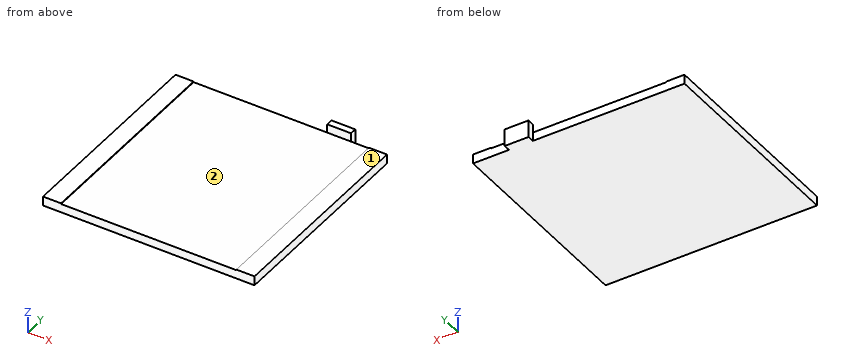
from build123d import *

# Parameters (mm, degrees)
SKETCH1_W           = 159.25
SKETCH1_H           = 155.74
BOSS_EXTRUDE1_DEPTH = 6.5
SKETCH2_W           = 13.61
SKETCH2_H           = 155.74
BOSS_EXTRUDE2_DEPTH = 0.5
SKETCH3_W           = 17.92
SKETCH3_H           = 13
BOSS_EXTRUDE3_DEPTH = 5


with BuildPart() as part:
    # Sketch1 → Boss-Extrude1 (new body)
    with BuildSketch(Plane.XY):
        with Locations((79.625, 77.87)):
            Rectangle(SKETCH1_W, SKETCH1_H)
    extrude(amount=BOSS_EXTRUDE1_DEPTH)

    # Sketch2 → Boss-Extrude2 (add)
    with BuildSketch(Plane.XY.offset(6.5)):
        with Locations((6.805, 77.87)):
            Rectangle(SKETCH2_W, SKETCH2_H)
        with Locations((152.445, 77.87)):
            Rectangle(SKETCH2_W, SKETCH2_H)
    extrude(amount=BOSS_EXTRUDE2_DEPTH)

    # Sketch3 → Boss-Extrude3 (add)
    with BuildSketch(Plane(origin=(0, 155.74, 0), x_dir=(1, 0, 0), z_dir=(0, 1, 0))):
        with Locations((123.18, -6.5)):
            Rectangle(SKETCH3_W, SKETCH3_H)
    extrude(amount=BOSS_EXTRUDE3_DEPTH)


solid = part.part
Can you work these out from the model? Positions are in its coordinate system, mm. Face numbers are marked on the shaded views. Give positions to 0.01 mm unless a question says otherwise; leave off trailing zeros. Order: outer loops, then holes, each group sorted by start corner. A loop starts at its lowest first (then second) coordinate and runs counter-clockwise, first axis right, second up. Notation, with made-up numbers: M 54,23.5 L 69,23.5 A27 cw 69,53.5 Z; hole C -39.5,19.5 d10. An arc over 180 degrees is marked long. Use one line per item in the form item = value. Start each with the question number.
Item 1: If we section it at A-A (y = 72): Write out the boundary of the cut face in (x, z), then the cut area to 3 significant figures.
Item 2: Will these pins go through, and if not, where does the flat tip stop? pin 1 Ø2 at (x, z) = (36, 5) entering from +Y; pin 2 Ø0.6 at (y, z) = (68, 6.5) entering from -X; pin 3 Ø7 at (x, y) = (152, 60) entering from +Z; pin 4 Ø12 at (x, y) = (118, 112.5) entering from +Z.
Item 3: If I drill on line 1 along Y through (x, z) = (26, 6.25); line 2 along Z through (x, y) = (23.5, 22); line 3 along Z through (x, y) = (10, 90.5), over which ranges is the centre line in solid material (lowest first)?
Item 4: If we section it at D-D (x = 134.5): Write out the boundary of the cut face in (y, z), then the cut area to 3 significant figures.
Item 5: We'd pull the mould along X, two halves only. Please class the marked faces 1 and 2: +X half, -X half, draft (parallel to the pull), parting line (faces both ways), or undercut.
Item 6: If we section it at C-C (z = 4.5): Write out the boundary of the cut face in (x, y).
Item 7: If we section it at B-B (x = 118): Write out the boundary of the cut face in (y, z).
Outcome:
q1.outline = M 0,0 L 159.25,0 L 159.25,7 L 145.64,7 L 145.64,6.5 L 13.61,6.5 L 13.61,7 L 0,7 Z
q1.area = 1,050 mm2
q2.pin_1 = 155.74
q2.pin_2 = 0
q2.pin_3 = 7
q2.pin_4 = 6.5
q3.line_1 = 0 to 155.74
q3.line_2 = 0 to 6.5
q3.line_3 = 0 to 7
q4.outline = M 0,0 L 155.74,0 L 155.74,6.5 L 0,6.5 Z
q4.area = 1,010 mm2
q5.face_1 = draft
q5.face_2 = undercut
q6.outline = M 0,0 L 159.25,0 L 159.25,155.74 L 132.14,155.74 L 132.14,160.74 L 114.22,160.74 L 114.22,155.74 L 0,155.74 Z
q7.outline = M 0,0 L 160.74,0 L 160.74,13 L 155.74,13 L 155.74,6.5 L 0,6.5 Z
